Design review of the part built by this model. Coordinates are the model's own, in mm. Face numbers are marked on the shaded views. A direction names the side the tool comes from. Give positions to 0.01 mm unless a question says otherwise; leave off trailing zeros. Loops run counter-clockwise (first coordinate to the right, second up) from the corner with the lowest first, then second, coordinate; pieces in that order, holes last. Notation, with made-up numbers: (-24, -36) - (4, -36) arc R32 cw to (4, -6) - close; hole circle Ø2 at (-40, 8.25). An arc over 180 degrees is marked (long way). One line per item, written item: value. Start each with the question number.
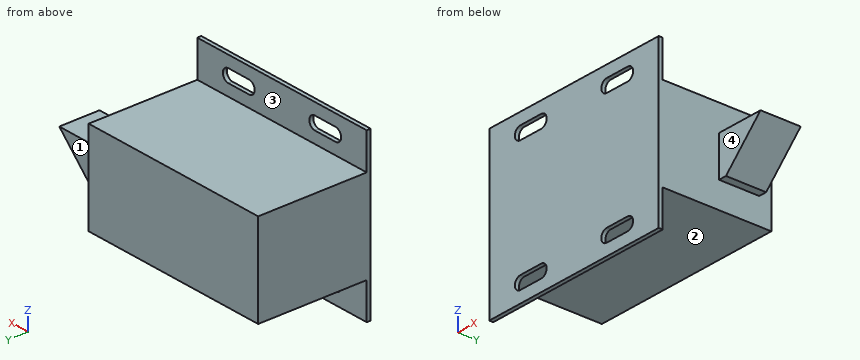
```python
from build123d import *

# Parameters (mm, degrees)
SKETCH1_W           = 49
SKETCH1_H           = 41
BOSS_EXTRUDE1_DEPTH = 1
SKETCH2_W           = 49
SKETCH2_H           = 23
BOSS_EXTRUDE2_DEPTH = 27
SKETCH3_W           = 10
SKETCH3_H           = 10
BOSS_EXTRUDE3_DEPTH = 12
CHAMFER1_SIZE       = 10


with BuildPart() as part:
    # Sketch1 → Boss-Extrude1 (new body)
    with BuildSketch(Plane(origin=(0, 0, 0), x_dir=(1, 0, 0), z_dir=(0, 1, 0))):
        with Locations((24.5, 20.5)):
            Rectangle(SKETCH1_W, SKETCH1_H)
        with BuildLine():
            Line((9, 38.1), (15, 38.1))
            ThreePointArc((15, 38.1), (16.6, 36.5), (15, 34.9))
            Line((15, 34.9), (9, 34.9))
            ThreePointArc((9, 34.9), (7.4, 36.5), (9, 38.1))
        make_face(mode=Mode.SUBTRACT)
        with BuildLine():
            Line((34, 38.1), (40, 38.1))
            ThreePointArc((40, 38.1), (41.6, 36.5), (40, 34.9))
            Line((40, 34.9), (34, 34.9))
            ThreePointArc((34, 34.9), (32.4, 36.5), (34, 38.1))
        make_face(mode=Mode.SUBTRACT)
        with BuildLine():
            Line((34, 6.1), (40, 6.1))
            ThreePointArc((40, 6.1), (41.6, 4.5), (40, 2.9))
            Line((40, 2.9), (34, 2.9))
            ThreePointArc((34, 2.9), (32.4, 4.5), (34, 6.1))
        make_face(mode=Mode.SUBTRACT)
        with BuildLine():
            Line((15, 2.9), (9, 2.9))
            ThreePointArc((9, 2.9), (7.4, 4.5), (9, 6.1))
            Line((9, 6.1), (15, 6.1))
            ThreePointArc((15, 6.1), (16.6, 4.5), (15, 2.9))
        make_face(mode=Mode.SUBTRACT)
    extrude(amount=BOSS_EXTRUDE1_DEPTH)

    # Sketch2 → Boss-Extrude2 (add)
    with BuildSketch(Plane(origin=(0, 1, 0), x_dir=(1, 0, 0), z_dir=(0, 1, 0))):
        with Locations((24.5, 20.5)):
            Rectangle(SKETCH2_W, SKETCH2_H)
    extrude(amount=BOSS_EXTRUDE2_DEPTH)

    # Sketch3 → Boss-Extrude3 (add)
    with BuildSketch(Plane(origin=(49, 0, 0), x_dir=(0, 0, -1), z_dir=(1, 0, 0))):
        with Locations((20.5, 20)):
            Rectangle(SKETCH3_W, SKETCH3_H)
    extrude(amount=BOSS_EXTRUDE3_DEPTH)

    # Chamfer1
    chamfer1_edges = [part.edges().sort_by_distance(p)[0] for p in [
        (61, 20, -25.5),
    ]]
    chamfer(chamfer1_edges, length=CHAMFER1_SIZE - 0.0001)  # a hair under: the kernel refuses the full size


solid = part.part
```
(1) To check wall thickness, follow L1, parallel to Z at x = 19.5, y = 19.5; L2, parallel to Y at x = 19.5, z = -4.5; L3, parallel to X at y = 11, z = -23. State the ranges of each line that lie inside material, in increasing order. Write a range as from..to.
(2) Machinability: for the marked faces 1, 2, 3 and 4, which of the approach directions +Z, -Z, +X, -X, +Y, -Y give a long, thin tool a straight path to every point of the face, cutting with its end or side? Answer none if there is none.
(3) Take a section at D-D on z = -22.5. State the section outline as (x, y) points, and give its area (3 significant figures).
(4) Take a section at A-A on z = -4.5. State the section outline as (x, y) points, and give its area (3 significant figures).
(5) Take a section at C-C on x = 23. State the section outline as (y, z) points, and give its area (3 significant figures).
(6) For pin 1 Ø1.5 at (y, z) = (4, -26.5) entering from +X; pin 2 Ø0.8 at (x, y) = (11, 0.5) entering from +Z; pin 3 Ø2 at (x, y) = (19.5, 23.5) entering from -Z; pin 4 Ø11 at (x, z) = (57.5, -19.5) entering from +Y, all flat-tipped, find the tip position at first contact; note any pin that passes through.
Here are the results:
1. L1: -32..-9
1. L2: 0..1
1. L3: 0..49
2. face 1: +Z, -Z, +X, +Y
2. face 2: -Z, +X, -X, +Y
2. face 3: +Z, +X, -X, +Y
2. face 4: +Z, -Z, +X, -Y
3. outline: (0, 0) - (49, 0) - (49, 15) - (54, 15) - (54, 25) - (49, 25) - (49, 28) - (0, 28) - close
3. area: 1,420 mm²
4. outline: (0, 0) - (7.4, 0) - (7.4, 1) - (0, 1) - close; (16.6, 0) - (32.4, 0) - (32.4, 1) - (16.6, 1) - close; (41.6, 0) - (49, 0) - (49, 1) - (41.6, 1) - close
4. area: 30.6 mm²
5. outline: (0, -41) - (1, -41) - (1, -32) - (28, -32) - (28, -9) - (1, -9) - (1, 0) - (0, 0) - close
5. area: 662 mm²
6. pin 1: x = 49
6. pin 2: z = 0
6. pin 3: z = -32
6. pin 4: y = 25
